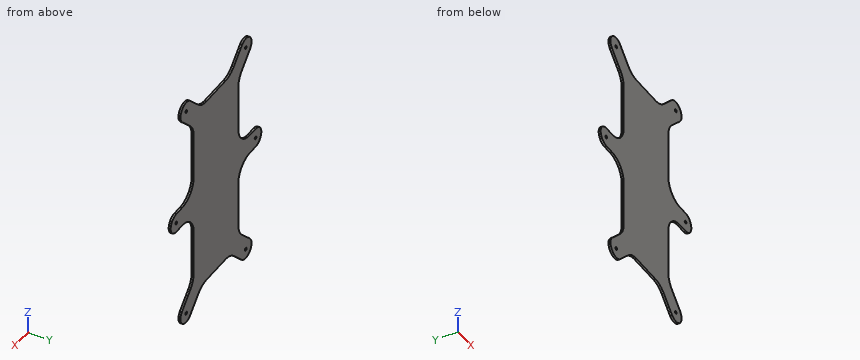
from build123d import *

# Parameters (mm, degrees)
EXTRUDE_1_DEPTH       = 2
CUT_EXTRUDE_1_DEPTH   = 147.138709345
MIRROR_2_COPY_1_DEPTH = 147.138709345
FILLET_1_R            = 20
SKETCH_4_R            = 1.5
CUT_EXTRUDE_2_DEPTH   = 147.138709345


with BuildPart() as part:
    # 草图2 → 凸台-拉伸1 (new body)
    with BuildSketch(Plane(origin=(0, 0, 0), x_dir=(1, 0, 0), z_dir=(0, 1, 0))):
        with BuildLine():
            Line((-69, -10), (-59, -10))
            ThreePointArc((-59, -10), (-44.857864376, -15.857864376), (-39, -30))
            Line((-39, -30), (-39, -73.141444367))
            ThreePointArc((-39, -73.141444367), (-40.081491111, -79.629126652), (-43.209002143, -85.415171865))
            Line((-43.209002143, -85.415171865), (-59.824431116, -106.792068439))
            ThreePointArc((-59.824431116, -106.792068439), (-59, -120), (-45.792068439, -120.824431116))
            Line((-45.792068439, -120.824431116), (-24.415171865, -104.209002143))
            ThreePointArc((-24.415171865, -104.209002143), (-18.629126652, -101.081491111), (-12.141444367, -100))
            Line((-12.141444367, -100), (12.141444367, -100))
            ThreePointArc((12.141444367, -100), (18.629126652, -101.081491111), (24.415171865, -104.209002143))
            Line((24.415171865, -104.209002143), (45.792068439, -120.824431116))
            ThreePointArc((45.792068439, -120.824431116), (59, -120), (59.824431116, -106.792068439))
            Line((59.824431116, -106.792068439), (43.209002143, -85.415171865))
            ThreePointArc((43.209002143, -85.415171865), (40.081491111, -79.629126652), (39, -73.141444367))
            Line((39, -73.141444367), (39, -30))
            ThreePointArc((39, -30), (44.857864376, -15.857864376), (59, -10))
            Line((59, -10), (69, -10))
            ThreePointArc((69, -10), (79, 0), (69, 10))
            Line((69, 10), (59, 10))
            ThreePointArc((59, 10), (44.857864376, 15.857864376), (39, 30))
            Line((39, 30), (39, 73.141444367))
            ThreePointArc((39, 73.141444367), (40.081491111, 79.629126652), (43.209002143, 85.415171865))
            Line((43.209002143, 85.415171865), (59.824431116, 106.792068439))
            ThreePointArc((59.824431116, 106.792068439), (59, 120), (45.792068439, 120.824431116))
            Line((45.792068439, 120.824431116), (24.415171865, 104.209002143))
            ThreePointArc((24.415171865, 104.209002143), (18.629126652, 101.081491111), (12.141444367, 100))
            Line((12.141444367, 100), (-12.141444367, 100))
            ThreePointArc((-12.141444367, 100), (-18.629126652, 101.081491111), (-24.415171865, 104.209002143))
            Line((-24.415171865, 104.209002143), (-45.792068439, 120.824431116))
            ThreePointArc((-45.792068439, 120.824431116), (-59, 120), (-59.824431116, 106.792068439))
            Line((-59.824431116, 106.792068439), (-43.209002143, 85.415171865))
            ThreePointArc((-43.209002143, 85.415171865), (-40.081491111, 79.629126652), (-39, 73.141444367))
            Line((-39, 73.141444367), (-39, 30))
            ThreePointArc((-39, 30), (-44.857864376, 15.857864376), (-59, 10))
            Line((-59, 10), (-69, 10))
            ThreePointArc((-69, 10), (-79, 0), (-69, -10))
        make_face()
    extrude(amount=EXTRUDE_1_DEPTH)

    # 草图3 → 切除-拉伸1 (cut, through all)
    with BuildSketch(Plane(origin=(0, 2, 0), x_dir=(1, 0, 0), z_dir=(0, 1, 0))):
        Polygon((24.857864376, 100), (12.141444367, 100), (45.299236161, 120.441371785), align=None)
        Polygon((39, 73.141444367), (59.441371785, 106.299236161), (39, 85.857864376), align=None)
    cut_extrude_1 = extrude(amount=-CUT_EXTRUDE_1_DEPTH, mode=Mode.SUBTRACT)

    # 镜向1: 切除-拉伸1 across plane
    add(cut_extrude_1.mirror(Plane.XY), mode=Mode.SUBTRACT)

    # 镜向2: 切除-拉伸1 across plane
    add(cut_extrude_1.mirror(Plane(origin=(0, 0, 0), x_dir=(0, 0, 1), z_dir=(1, 0, 0))), mode=Mode.SUBTRACT)

    # 镜向2 copy 1 sketch → 镜向2 copy 1 (cut, through all)
    with BuildSketch(Plane(origin=(0, 2, 0), x_dir=(-1, 0, 0), z_dir=(0, 1, 0))):
        Polygon((24.857864376, 100), (12.141444367, 100), (45.299236161, 120.441371785), align=None)
        Polygon((39, 73.141444367), (59.441371785, 106.299236161), (39, 85.857864376), align=None)
    extrude(amount=-MIRROR_2_COPY_1_DEPTH, mode=Mode.SUBTRACT)

    # 圆角1
    fillet_1_edges = [part.edges().sort_by_distance(p)[0] for p in [
        (39, 1, -85.857864376),
        (24.857864376, 1, -100),
        (39, 1, 85.857864376),
        (24.857864376, 1, 100),
        (-39, 1, -85.857864376),
        (-24.857864376, 1, -100),
        (-39, 1, 85.857864376),
        (-24.857864376, 1, 100),
    ]]
    fillet(fillet_1_edges, radius=FILLET_1_R)

    # 草图4 → 切除-拉伸2 (cut, through all)
    with BuildSketch(Plane(origin=(0, 2, 0), x_dir=(1, 0, 0), z_dir=(0, 1, 0))):
        with Locations(Location((69, 0, 0), (0, 0, 270))):
            Circle(SKETCH_4_R)
        with Locations(Location((51.928932188, 112.928932188, 0), (0, 0, 270))):
            Circle(SKETCH_4_R)
        with Locations(Location((51.928932188, -112.928932188, 0), (0, 0, 90))):
            Circle(SKETCH_4_R)
        with Locations(Location((-69, 0, 0), (0, 0, 90))):
            Circle(SKETCH_4_R)
        with Locations(Location((-51.928932188, 112.928932188, 0), (0, 0, 90))):
            Circle(SKETCH_4_R)
        with Locations(Location((-51.928932188, -112.928932188, 0), (0, 0, 270))):
            Circle(SKETCH_4_R)
    extrude(amount=-CUT_EXTRUDE_2_DEPTH, mode=Mode.SUBTRACT)


solid = part.part
Work out the finished part from the listing and answer in its coordinate system (mm). Round coordinates to 2 decimals unless told otherwise and drop trailing zeros. Write each loop counter-clockwise with the first axis right and the second up, starting at its lowest first coordinate (ties: lowest second). Pieces come first, ordered by that corner, then holes. Notation, with made-up numbers: M 7.5,29.5 L 44.5,29.5 A21 ccw 44.5,55.5 Z; hole C -33.5,14 d1. An arc over 180 degrees is marked long. Use a Markdown table: item, result.
1) The part is cut by section A-A on x = 8. Give the vertices of the cut face in (y, z).
Taken from the geometry:
| item | result |
|---|---|
| outline | M 0,-100 L 2,-100 L 2,100 L 0,100 Z |
2) Consider line 1 (X direction, y = 1.2, z = 0); line 2 (Z direction, x = 42, y = 0.35); line 3 (Z direction, x = 69, y = 1.05). Determine where each line is inside the solid, lowest interval first. Write a range as [from, to].
Taken from the geometry:
| item | result |
|---|---|
| line 1 | x = [-79, -70.5], [-67.5, 67.5], [70.5, 79] |
| line 2 | z = [-117.14, -88.11], [-19.46, 19.46], [88.11, 117.14] |
| line 3 | z = [-10, -1.5], [1.5, 10] |
3) The part is cut by section C-C on y = 0.3. State how many separate pieces and enclosed holes the cut face has, plus the area to 3 significant figures.
Taken from the geometry:
| item | result |
|---|---|
| separate pieces | 1 |
| enclosed holes | 6 |
| area | 20,000 mm2 |
4) The part is cut by section B-B on z = -48. Give the vertices of the cut face in (x, y).
Taken from the geometry:
| item | result |
|---|---|
| outline | M -39,0 L 39,0 L 39,2 L -39,2 Z |
